For this review, take the finished solid that the model builds, in its own axes (mm). Give positions to 0.01 mm unless a question says otherwise; leave off trailing zeros. Order: outer loops, then holes, each group sorted by start corner. A loop starts at its lowest first (then second) coordinate and runs counter-clockwise, first axis right, second up. Notation, with made-up numbers: (-39, -14.75) -> (10, -14.75) arc R22 cw to (10, 21.25) -> close; hole circle Ø6 at (-7.75, -14). An arc over 180 degrees is marked (long way). Return JSON: item names as keys, results as strings. Group by question number.
1) The part is to be moulded in two halves that separate along Z. For faces 1 (the face through (0.275, -3.527, 2.019)), 2 (the face through (0.275, -0.388, 1.748)), 3 (the face through (0, -2, 0)), say which applies: released by +Z, released by -Z, zero draft, split by the parting line, or undercut.
2) Add section C-C (z = -3.5). Give the boundary of the cut face in (x, y), then the cut area to 3 significant figures.
3) Insertion check: P1, Ø4, axis at y = 0, z = 0, coming from the +X side. The pin has a flat end and moves straight along its axis. Give the tip position at first contact, or say it passes through.
4) Add section B-B (y = 0). Give the boundary of the cut face in (x, z).
5) To check wall thickness, follow line 1 along Z through (x, y) = (0.2, 0); line 2 along Z through (x, y) = (0.45, 3); line 3 along Y through (x, z) = (0.2, -1.5). State the ranges of each line that lie inside material, in increasing order.
6) Add section D-D (y = -2.75). Give the boundary of the cut face in (x, z).
7) Add section A-A (z = 0). Give the boundary of the cut face in (x, y).
Autodesk Inventor part; units mm, degrees
ref_plane "Work Plane1" through (0, 0, 0) normal (0, -1, 0) x (1, 0, 0)
ref_plane "YZ Plane" through (0, 0, 0) normal (1, 0, 0) x (0, 1, 0)
ref_plane "XZ Plane" through (0, 0, 0) normal (0, 1, 0) x (-1, 0, 0)
sketch "Sketch1" plane through (0, 0, 0) normal (1, 0, 0) x (0, 1, 0)
  circle A0 centre (0, 0) radius 4.064
  circle A1 centre (0, 0) radius 1.7907
  dimension "d0" = 8.128
  dimension "d1" = 3.5814
extrude "Body" add sketch "Sketch1" along normal blind 0.5588
sketch "Sketch2" plane through (0.5588, 0, 0) normal (1, 0, 0) x (0, 0, -1)
  circle A0 centre (0, 0) radius 4.064
  line L0 (0, 0) -> (0, 4.064) construction
  arc A1 (1.0518, 3.9255) -> (-1.0518, 3.9255) centre (0, 0) ccw
  arc A2 (0.7577, 2.8276) -> (-0.7577, 2.8276) centre (0, 0) ccw
  line L1 (-0.7577, 2.8276) -> (-1.0518, 3.9255)
  line L2 (0.7577, 2.8276) -> (1.0518, 3.9255)
  line L3 (-0.7577, 2.8276) -> (0, 0) construction
  line L4 (0, 0) -> (0.7577, 2.8276) construction
  dimension "d4" = 30
  dimension "d5" = 5.8547
extrude "Cut" cut sketch "Sketch2" against normal through all contours L2 A2 L1 A0 picked at (0.0851, 3.6711)
fillet "Fillet1" radius 0.1219 2 edges at (0.2794, 2.8276, 0.7577) (0.2794, 2.8276, -0.7577)
pattern_circular "Cuts" count 6 over 360 about axis through (0, 0, 0) along (1, 0, 0) of "Cut", "Fillet1"
ref_plane "Work Plane1" through (0, 0, 0) normal (0, -1, 0) x (1, 0, 0)
equation "\"d0\" = SD2"
equation "\"d1\" = SD1"
equation "\"d2\" = SD"
equation "\"d5\" = 0.5 * SD2 + 0.5 * SD1"
equation "\"d6\" = SD"
equation "\"d8\" = 0.015 * SD2"
equation "\"SD\" = 0.5588"
equation "\"SD1\" = 3.5814"
equation "\"SD2\" = 8.128"
equation "\"NND\" = 3.5052"
properties part number "ASME B18.21.1 - No. 6. Carbon Steel" material "Steel, Mild"
Evaluation:
{
 "1": {"face 1": "released by +Z", "face 2": "undercut", "face 3": "zero draft"},
 "2": {"outline": "(0, -0.94) -> (0.56, -0.94) -> (0.56, 0.94) -> (0, 0.94) -> close", "area": "1.05 mm^2"},
 "3": {"P1": "x = 0.56"},
 "4": {"outline": "(0, -4.06) -> (0.56, -4.06) -> (0.56, -1.79) -> (0, -1.79) -> close; (0, 1.79) -> (0.56, 1.79) -> (0.56, 4.06) -> (0, 4.06) -> close"},
 "5": {"line 1": "-4.06 to -1.79, 1.79 to 4.06", "line 2": "-2.74 to -0.8, 0.8 to 2.74", "line 3": "-3.78 to -0.98, 0.98 to 3.78"},
 "6": {"outline": "(0, -2.75) -> (0.56, -2.75) -> (0.56, 2.75) -> (0, 2.75) -> close"},
 "7": {"outline": "(0, -2.93) -> (0.56, -2.93) -> (0.56, -1.79) -> (0, -1.79) -> close; (0, 1.79) -> (0.56, 1.79) -> (0.56, 2.93) -> (0, 2.93) -> close"}
}
